Geometry: see drawing. Coordinates: mm, zero at the bounding-box minimum. A direction names the side the tool comes from. Give positions to 0.01 mm unless a question says otherwise; leave off trailing zeros. Write each loop counter-clockwise with the first axis right and the second up, starting at its lowest first coordinate (ties: lowest second). Pieces come first, ordered by that corner, then holes. Notation, with made-up numbers: M 55,29 L 89,29 A21 ccw 89,60 Z; hole C -26,-20.75 d3. An arc over 180 degrees is marked long. Use a Markdown table: item, result. Add a question column.
1) Section B-B on y = 3.5. Return the cut outline in (x, z).
2) Line query: line 1 (Z direction, x = 2.5, y = 3.4); line 2 (X direction, y = 3.8, z = 3.5); line 3 (Z direction, x = 2.5, y = 2.7). Output: solid intervals per line, ascending.
3) Pin query (flat end, axial travel): pin 1 (1 mm diameter, centred on x = 20, z = 5.5, fed in from +Y); pin 2 (1.7 mm diameter, centred on x = 6.5, z = 4, fed in from +Y); pin 3 (1.7 mm diameter, centred on y = 0.5, z = 3.5, fed in from -X). Return the tip coordinate at first contact, or that it passes through.
4) Set-up query: the marked faces 5, 6 and 7. Return all of +Z, -Z, +X, -X, +Y, -Y with unobstructed straight access to the full face (end or side cutting, diameter ignored); none if empty.
5) Section C-C on x = 4. Return the cut outline in (y, z), then the cut area to 3 significant figures.
6) Section D-D on x = 17. Return the cut outline in (y, z), then the cut area to 3 significant figures.
7) Section A-A on z = 3.5. Return the cut outline in (x, y).
8) Draft query along X for the marked faces 1, 2, 3 and 4. Return one class per face: +X half, -X half, draft (parallel to the pull), parting line (faces both ways), or undercut.
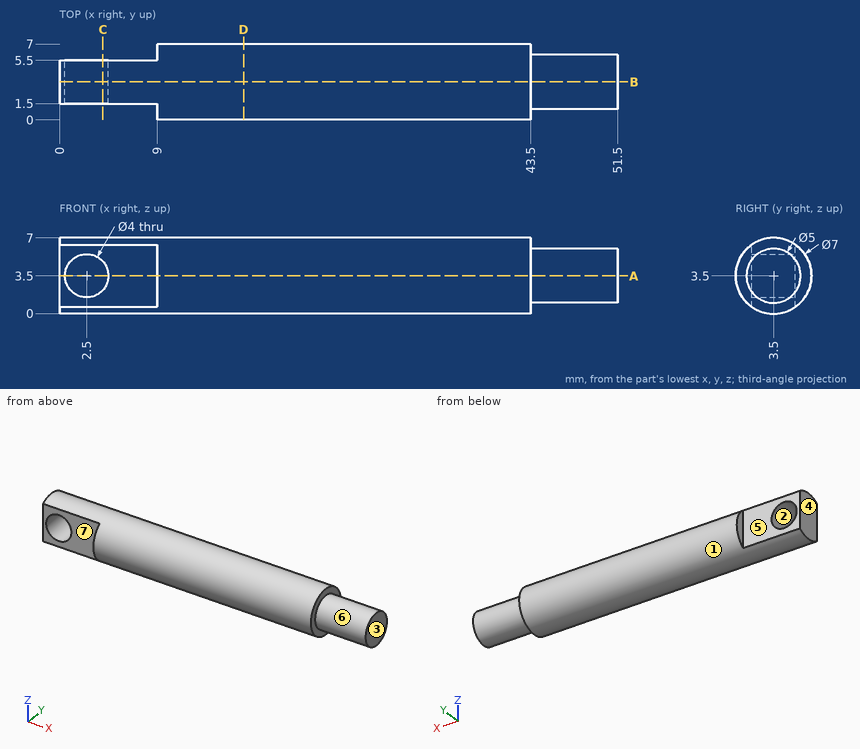
Found:
| question | item | result |
|---|---|---|
| 1 | outline | M 0,0 L 43.5,0 L 43.5,1 L 51.5,1 L 51.5,6 L 43.5,6 L 43.5,7 L 0,7 Z; hole C 2.5,3.5 d4 |
| 2 | line 1 | 0 to 1.5, 5.5 to 7 |
| 2 | line 2 | 0 to 0.5, 4.5 to 51.5 |
| 2 | line 3 | 0.09 to 1.5, 5.5 to 6.91 |
| 3 | pin 1 | y = 6.66 |
| 3 | pin 2 | y = 5.5 |
| 3 | pin 3 | x = 9 |
| 4 | face 5 | +Z, -Z, -X, +Y |
| 4 | face 6 | +X |
| 4 | face 7 | +Z, -Z, -X, -Y |
| 5 | outline | M 1.5,0.63 A3.5 ccw 5.5,0.63 L 5.5,2.18 L 1.5,2.18 Z; M 1.5,4.82 L 5.5,4.82 L 5.5,6.37 A3.5 ccw 1.5,6.37 Z |
| 5 | area | 15.8 mm² |
| 6 | outline | C 3.5,3.5 d7 |
| 6 | area | 38.5 mm² |
| 7 | outline | M 0,1.5 L 0.5,1.5 L 0.5,5.5 L 0,5.5 Z; M 4.5,1.5 L 9,1.5 L 9,0 L 43.5,0 L 43.5,1 L 51.5,1 L 51.5,6 L 43.5,6 L 43.5,7 L 9,7 L 9,5.5 L 4.5,5.5 Z |
| 8 | face 1 | draft |
| 8 | face 2 | undercut |
| 8 | face 3 | +X half |
| 8 | face 4 | -X half |
